from build123d import *

# Parameters (mm, degrees)
F0_W     = 76.2
F0_H     = 19.05
F1_DEPTH = 406.4
F2_W     = 63.5
F2_H     = 12.7
F3_DEPTH = 19.05
F4_R     = 6.35
F5_W     = 63.5
F5_H     = 12.7
F6_DEPTH = 19.05
F7_R     = 3.175


with BuildPart() as f1:
    # F0 (on Front) → F1 (new body)
    with BuildSketch(Plane.XZ):
        with Locations((3.478697, 20.384602)):
            Rectangle(F0_W, F0_H)
    extrude(amount=-F1_DEPTH)

    # F2 (on face) → F3 (join)
    with BuildSketch(Plane.XZ):
        with Locations((3.478697, 20.384602)):
            Rectangle(F2_W, F2_H)
    extrude(amount=F3_DEPTH)

    # F4
    f4_edges = [f1.edges().sort_by_distance(p)[0] for p in [
        (41.578697, 203.2, 29.909602),
        (41.578697, 203.2, 10.859602),
        (-34.621303, 203.2, 29.909602),
        (-34.621303, 203.2, 10.859602),
    ]]
    fillet(f4_edges, radius=F4_R)

    # F5 (on face) → F6 (join)
    with BuildSketch(Plane(origin=(0, 406.4, 0), x_dir=(-1, 0, 0), z_dir=(0, 1, 0))):
        with Locations((-3.478697, 20.384602)):
            Rectangle(F5_W, F5_H)
    extrude(amount=F6_DEPTH)

    # F7
    f7_edges = [f1.edges().sort_by_distance(p)[0] for p in [
        (35.228697, -9.525, 26.734602),
        (35.228697, -9.525, 14.034602),
        (-28.271303, -9.525, 26.734602),
        (-28.271303, -9.525, 14.034602),
    ]]
    fillet(f7_edges, radius=F7_R)


solid = f1.part
Could you check a few things on this model? Use its own coordinates, in mm. A direction names the side the tool comes from. Coordinates: 2 decimals unless noted, no trailing zeros. Order: outer loops, then holes, each group sorted by start corner. A loop starts at its lowest first (then second) coordinate and runs counter-clockwise, first axis right, second up. Notation, with made-up numbers: (26, -16.75) - (85, -16.75) arc R8 cw to (85, -7.75) - close; hole circle Ø9 at (-31.75, 29). An arc over 180 degrees is marked (long way). Answer in a Markdown table with one row per item. Add a question column.
(1) Will these pins go through, and if not, where does the flat tip stop? pin 1 (6.5 mm diameter, centred on y = 419.5, z = 18.5, fed in from +X); pin 2 (7 mm diameter, centred on y = -9.5, z = 21, fed in from -X); pin 3 (9.5 mm diameter, centred on x = 10, y = 412.5, fed in from -Z).
(2) I need wall thicknesses on L1, parallel to Y at x = 3, z = 12; L2, parallel to X at y = 228, z = 16.75; L3, parallel to X at y = 358, z = 28. Which ranges of each line are inside material? Lowest first, please.
(3) If we section it at B-B, the plane x = -11: Please give me the cut outline in (y, z).
(4) On a 3-axis mill with a long thin cutter (end or side, diameter ignored), from which of +Z, -Z, +X, -X, +Y, -Y can I reach the whole of each face in a straight line? I mean faces 1 (the face through (3, -9, 14.035)), 2 (the face through (4, 416, 14.035)), 3 (the face through (3, -9, 26.735)), 4 (the face through (35.229, 416, 20)). Say none if no direction works.
(5) If we section it at A-A, the plane y = 92.5: Please give me the cut outline in (x, z).
Results are:
| question | item | result |
|---|---|---|
| 1 | pin 1 | stops at x = 35.23 |
| 1 | pin 2 | stops at x = -28.27 |
| 1 | pin 3 | stops at z = 14.03 |
| 2 | L1 | y = 0 to 406.4 |
| 2 | L2 | x = -34.6 to 41.56 |
| 2 | L3 | x = -32.81 to 39.77 |
| 3 | outline | (-19.05, 14.03) - (0, 14.03) - (0, 10.86) - (406.4, 10.86) - (406.4, 14.03) - (425.45, 14.03) - (425.45, 26.73) - (406.4, 26.73) - (406.4, 29.91) - (0, 29.91) - (0, 26.73) - (-19.05, 26.73) - close |
| 4 | face 1 | -Z, +X, -X, -Y |
| 4 | face 2 | -Z, +X, -X, +Y |
| 4 | face 3 | +Z, +X, -X, -Y |
| 4 | face 4 | +Z, -Z, +X, +Y |
| 5 | outline | (-34.62, 17.21) arc R6.35 ccw to (-28.27, 10.86) - (35.23, 10.86) arc R6.35 ccw to (41.58, 17.21) - (41.58, 23.56) arc R6.35 ccw to (35.23, 29.91) - (-28.27, 29.91) arc R6.35 ccw to (-34.62, 23.56) - close |
